Verification items for the finished model (mm, model axes). A direction names the side the tool comes from. Give positions to 0.01 mm unless a question says otherwise; leave off trailing zeros. Write each loop counter-clockwise with the first axis right and the second up, starting at its lowest first coordinate (ties: lowest second). Pieces come first, ordered by that corner, then holes. Notation, with made-up numbers: (-27, -5.5) - (-12, -5.5) arc R21 ccw to (-12, 19.5) - close; hole circle Ø8 at (18.5, 70). An arc over 180 degrees is marked (long way). Put each result on its own line as item: value.
from build123d import *

# Parameters (mm, degrees)
SKETCH1_R           = 0.019660033
SKETCH1_R_2         = 1.5625
BOSS_EXTRUDE1_DEPTH = 2
FILLET1_R           = 1.5
SKETCH3_R           = 2
CUT_EXTRUDE2_DEPTH  = 37.527386986
CUT_EXTRUDE3_DEPTH  = 37.527386986


with BuildPart() as part:
    # Sketch1 → Boss-Extrude1 (new body)
    with BuildSketch(Plane.XY):
        with BuildLine():
            Line((-15, -32), (15, -32))
            ThreePointArc((15, -32), (16.767766953, -31.267766953), (17.5, -29.5))
            Line((17.5, -29.5), (17.5, 29.5))
            ThreePointArc((17.5, 29.5), (16.767766953, 31.267766953), (15, 32))
            Line((15, 32), (-15, 32))
            ThreePointArc((-15, 32), (-16.767766953, 31.267766953), (-17.5, 29.5))
            Line((-17.5, 29.5), (-17.5, -29.5))
            ThreePointArc((-17.5, -29.5), (-16.767766953, -31.267766953), (-15, -32))
        make_face()
        with Locations((-11.556302767, -27.879566704)):
            Circle(SKETCH1_R, mode=Mode.SUBTRACT)
        with Locations((-13.25, -26.25)):
            Circle(SKETCH1_R_2, mode=Mode.SUBTRACT)
        with Locations(Location((-13.25, 26.25, 0), (0, 0, 180))):
            Circle(SKETCH1_R_2, mode=Mode.SUBTRACT)
        with Locations(Location((13.25, -26.25, 0), (0, 0, 180))):
            Circle(SKETCH1_R_2, mode=Mode.SUBTRACT)
        with Locations((13.25, 26.25)):
            Circle(SKETCH1_R_2, mode=Mode.SUBTRACT)
    extrude(amount=BOSS_EXTRUDE1_DEPTH)

    # Fillet1
    fillet1_edges = [part.edges().sort_by_distance(p)[0] for p in [
        (16.767766953, -31.267766953, 2),
        (17.5, 0, 2),
        (16.767766953, 31.267766953, 2),
        (0, 32, 2),
        (-16.767766953, 31.267766953, 2),
        (-17.5, 0, 2),
        (-16.767766953, -31.267766953, 2),
        (0, -32, 2),
    ]]
    fillet(fillet1_edges, radius=FILLET1_R)

    # Sketch3 → Cut-Extrude2 (cut, through all)
    with BuildSketch(Plane.XY.offset(2)):
        with Locations((0, 15.9)):
            Circle(SKETCH3_R)
    extrude(amount=-CUT_EXTRUDE2_DEPTH, mode=Mode.SUBTRACT)

    # Sketch2 → Cut-Extrude3 (cut, through all)
    with BuildSketch(Plane.XY.offset(2)):
        with BuildLine():
            Line((-8.5, -16), (-8.5, 21.04))
            ThreePointArc((-8.5, 21.04), (-7.5, 22.04), (-6.5, 21.04))
            Line((-6.5, 21.04), (-6.5, -16))
            ThreePointArc((-6.5, -16), (-7.5, -17), (-8.5, -16))
        make_face()
        with BuildLine():
            Line((8.5, -16), (8.5, 21.04))
            ThreePointArc((8.5, 21.04), (7.5, 22.04), (6.5, 21.04))
            Line((6.5, 21.04), (6.5, -16))
            ThreePointArc((6.5, -16), (7.5, -17), (8.5, -16))
        make_face()
    extrude(amount=-CUT_EXTRUDE3_DEPTH, mode=Mode.SUBTRACT)


solid = part.part
Q1. Release check for a two-part mould opening along Y. For faces 3 (the face through (-7.52, 22.04, 1.01)), 4 (the face through (0, 0, 2)), 5 (the face through (0.21, -31.57, 1.55)) record: released by +Y, released by -Y, zero draft, split by the parting line, or undercut.
Answers follow:
face 3: undercut
face 4: zero draft
face 5: released by -Y
Q2. Scan lines: line 1 along X through (y, z) = (-3.5, 0.7); line 2 along Y through (x, z) = (-13.25, 1.35); line 3 along Y through (x, z) = (14.5, 1.25). Record each from-to range of solid material in increasing order.
Answers follow:
line 1: x = -17.49 to -8.5, -6.5 to 6.5, 8.5 to 17.49
line 2: y = -31.74 to -27.81, -24.69 to 24.69, 27.81 to 31.74
line 3: y = -31.8 to -27.19, -25.31 to 25.31, 27.19 to 31.8
Q3. Section check C-C, the plane y = -14. Record the cut outline in (x, z), plus the area to 3 significant figures.
Answers follow:
outline: (-17.5, 0) - (-8.5, 0) - (-8.5, 2) - (-16, 2) arc R1.5 ccw to (-17.5, 0.5) - close; (-6.5, 0) - (6.5, 0) - (6.5, 2) - (-6.5, 2) - close; (8.5, 0) - (17.5, 0) - (17.5, 0.5) arc R1.5 ccw to (16, 2) - (8.5, 2) - close
area: 61.0 mm2
Q4. Set-up check for faces 1 (the face through (-16.748, 31.287, 0.247)), 2 (the face through (6.5, 3, 1)): record each of +Z, -Z, +X, -X, +Y, -Y from which the full face is reachable in a straight line by a thin tool's end or side.
Answers follow:
face 1: +Z, -Z, -X, +Y
face 2: +Z, -Z
Q5. Go/stop test with flat-tipped pins: pin 1 Ø0.6 at (y, z) = (0.5, 1) entering from +X; pin 2 Ø1.9 at (x, y) = (-13.25, 26.25) entering from +Z. Record where each tip stops, or that it passes through.
Answers follow:
pin 1: stops at x = 17.49
pin 2: passes through
Q6. Section check B-B, the plane x = 7.5. Record the cut outline in (y, z).
Answers follow:
outline: (-32, 0) - (-17, 0) - (-17, 2) - (-30.5, 2) arc R1.5 ccw to (-32, 0.5) - close; (22.04, 0) - (32, 0) - (32, 0.5) arc R1.5 ccw to (30.5, 2) - (22.04, 2) - close
Q7. Section check D-D, the plane x = 13.25. Record the cut outline in (y, z), plus the area to 3 significant figures.
Answers follow:
outline: (-32, 0) - (-27.81, 0) - (-27.81, 2) - (-30.5, 2) arc R1.5 ccw to (-32, 0.5) - close; (-24.69, 0) - (24.69, 0) - (24.69, 2) - (-24.69, 2) - close; (27.81, 0) - (32, 0) - (32, 0.5) arc R1.5 ccw to (30.5, 2) - (27.81, 2) - close
area: 115 mm2
Q8. Section check A-A, the plane y = 15.9. Record the cut outline in (x, z).
Answers follow:
outline: (-17.5, 0) - (-8.5, 0) - (-8.5, 2) - (-16, 2) arc R1.5 ccw to (-17.5, 0.5) - close; (-6.5, 0) - (-2, 0) - (-2, 2) - (-6.5, 2) - close; (2, 0) - (6.5, 0) - (6.5, 2) - (2, 2) - close; (8.5, 0) - (17.5, 0) - (17.5, 0.5) arc R1.5 ccw to (16, 2) - (8.5, 2) - close
